Check sheet for the modelled part. Datum: model origin and axes. Units: mm. A direction names the side the tool comes from. Give positions to 0.01 mm unless a question says otherwise; leave off trailing zeros. Order: outer loops, then holes, each group sorted by start corner. A loop starts at its lowest first (then second) coordinate and runs counter-clockwise, first axis right, second up. Notation, with made-up numbers: M 36,-12.75 L 92,-12.75 A25 cw 92,21.25 Z; hole C -16,-5 d3. An arc over 180 degrees is marked long. Answer in a Markdown table with one row per item. Add a question column.
from build123d import *

# Parameters (mm, degrees)
SKETCH1_W           = 95
SKETCH1_H           = 150
SKETCH1_R           = 2
SKETCH1_R_2         = 26
SKETCH1_W_2         = 60
SKETCH1_H_2         = 10
BOSS_EXTRUDE1_DEPTH = 10
FILLET1_R           = 10


with BuildPart() as part:
    # Sketch1 → Boss-Extrude1 (new body)
    # profile 1 of 2: a face of its own
    with BuildSketch(Plane.XY):
        with Locations((0, 23)):
            Rectangle(SKETCH1_W, SKETCH1_H)
        with Locations((-26.846787517, 15.5)):
            Circle(SKETCH1_R, mode=Mode.SUBTRACT)
        with Locations((-26.846787517, -15.5)):
            Circle(SKETCH1_R, mode=Mode.SUBTRACT)
        with Locations((0, -31)):
            Circle(SKETCH1_R, mode=Mode.SUBTRACT)
        with Locations((26.846787517, -15.5)):
            Circle(SKETCH1_R, mode=Mode.SUBTRACT)
        with Locations((26.846787517, 15.5)):
            Circle(SKETCH1_R, mode=Mode.SUBTRACT)
        with Locations((0, 31)):
            Circle(SKETCH1_R, mode=Mode.SUBTRACT)
        Circle(SKETCH1_R_2, mode=Mode.SUBTRACT)
    # profile 2 of 2: a face of its own
    with BuildSketch(Plane.XY):
        with Locations((0, -57)):
            Rectangle(SKETCH1_W_2, SKETCH1_H_2)
    extrude(amount=BOSS_EXTRUDE1_DEPTH)

    # Fillet1
    fillet1_edges = [part.edges().sort_by_distance(p)[0] for p in [
        (-47.5, 98, 5),
        (47.5, 98, 5),
    ]]
    fillet(fillet1_edges, radius=FILLET1_R)


solid = part.part
Q1. Cross-section at A-A (y = 31). Record the boundary of the cut face in (x, z).
Q2. Tool access check on faces 1 (the flat face through (30, -57, 5)), 2 (the cylindrical face through (0, 29, 5)), 3 (the flat face through (-30, -57, 5)). Record the directions out of +Z, -Z, +X, -X, +Y, -Y that give a thin tool (end or side, any length) a straight path to the whole face; none if there is none.
Q3. Thickness scan on probe 1 along Y at (x, z) = (0, 4.25); probe 2 along Y at (x, z) = (36, 1.5); probe 3 along Y at (x, z) = (-9.5, 5.5). Record the ranges inside material, lowest first.
Q4. Go/stop test with flat-tipped pins: pin 1 (3 mm diameter, centred on x = 26.85, y = 15.5, fed in from +Z); pin 2 (3 mm diameter, centred on x = -42.5, z = 4.5, fed in from -Y); pin 3 (6.5 mm diameter, centred on x = -26.85, y = -15.5, fed in from +Z). Record where each tip stops, or that it passes through.
Q5. Cross-section at C-C (x = 0). Record the boundary of the cut face in (y, z), and give its area (3 significant figures).
Q6. Cross-section at B-B (z = 6). Record the boundary of the cut face in (x, y), and give its area (3 significant figures).
Q7. Cross-section at D-D (y = -15.5). Record the boundary of the cut face in (x, z), and give its area (3 significant figures).
Q8. Draft check along Y on faces 4 (the flat face through (-47.5, 17, 5)), 5 (the flat face through (-39, -52, 5)), 6 (the cylindrical face through (-20.633, -15.821, 4.93)), 7 (the cylindrical face through (25.37, -14.15, 4.93)). Enter one of: pulls with the +Y half, pulls with the -Y half, needs draft (parallel to the pull), parting line crosses it, or undercut.
Values follow:
| question | item | result |
|---|---|---|
| 1 | outline | M -47.5,0 L -2,0 L -2,10 L -47.5,10 Z; M 2,0 L 47.5,0 L 47.5,10 L 2,10 Z |
| 2 | face 1 | +Z, -Z, +X, -Y |
| 2 | face 2 | +Z, -Z |
| 2 | face 3 | +Z, -Z, -X, -Y |
| 3 | probe 1 | -62 to -33, -29 to -26, 26 to 29, 33 to 98 |
| 3 | probe 2 | -52 to 98 |
| 3 | probe 3 | -62 to -24.2, 24.2 to 98 |
| 4 | pin 1 | through |
| 4 | pin 2 | y = -52 |
| 4 | pin 3 | z = 10 |
| 5 | outline | M -62,0 L -33,0 L -33,10 L -62,10 Z; M -29,0 L -26,0 L -26,10 L -29,10 Z; M 26,0 L 29,0 L 29,10 L 26,10 Z; M 33,0 L 98,0 L 98,10 L 33,10 Z |
| 5 | area | 1,000 mm² |
| 6 | outline | M -47.5,-52 L -30,-52 L -30,-62 L 30,-62 L 30,-52 L 47.5,-52 L 47.5,88 A10 ccw 37.5,98 L -37.5,98 A10 ccw -47.5,88 Z; hole C -26.85,-15.5 d4; hole C -26.85,15.5 d4; hole C 0,0 d52; hole C 0,-31 d4; hole C 0,31 d4; hole C 26.85,-15.5 d4; hole C 26.85,15.5 d4 |
| 6 | area | 12,600 mm² |
| 7 | outline | M -47.5,0 L -28.85,0 L -28.85,10 L -47.5,10 Z; M -24.85,0 L -20.87,0 L -20.87,10 L -24.85,10 Z; M 20.87,0 L 24.85,0 L 24.85,10 L 20.87,10 Z; M 28.85,0 L 47.5,0 L 47.5,10 L 28.85,10 Z |
| 7 | area | 453 mm² |
| 8 | face 4 | needs draft |
| 8 | face 5 | pulls with the -Y half |
| 8 | face 6 | undercut |
| 8 | face 7 | undercut |
